Check sheet for the modelled part. Datum: model origin and axes. Units: mm. Coordinates: 2 decimals unless noted, no trailing zeros. Order: outer loops, then holes, each group sorted by start corner. A loop starts at its lowest first (then second) coordinate and runs counter-clockwise, first axis right, second up.
Autodesk Inventor part; units mm, degrees
ref_plane "YZ Plane" through (0, 0, 0) normal (1, 0, 0) x (0, 1, 0)
ref_plane "XZ Plane" through (0, 0, 0) normal (0, 1, 0) x (-1, 0, 0)
ref_plane "XY Plane" through (0, 0, 0) normal (0, 0, 1) x (1, 0, 0)
sketch "Sketch1" plane through (0, 0, 0) normal (1, 0, 0) x (0, 1, 0)
  line L0 (0, 80.1594) -> (0, -72.2406)
  circle A0 centre (101.6, 3.9594) radius 38.1
  line L1 (0, -72.2406) -> (114.2631, -31.9747)
  line L2 (0, 80.1594) -> (114.2631, 39.8934)
  point P0 (0, 0)
  dimension "d0" = 152.4
  dimension "d1" = 76.2
  dimension "d2" = 101.6
extrude "Extrusion1" add sketch "Sketch1" along normal blind 12.7
sketch "Sketch2" plane through (12.7, 0, 0) normal (1, 0, 0) x (0, 0, -1)
  arc A0 (31.9747, 114.2631) -> (-39.8934, 114.2631) centre (-3.9594, 101.6) ccw
  point P0 (0, 0)
hole "Hole1" at (12.7, 101.6, 3.9594) direction (-1, 0, 0) diameter 12.7 end through all
properties part number "Roller Frame"
(1) Cross-section at C-C (z = -11.5). Enter the section's corners in (x, y).
Filled in:
outline: (0, 0) - (12.7, 0) - (12.7, 136.42) - (0, 136.42) - close
(2) Go/stop test with flat-tipped pins: P1, Ø5, axis at x = 6, y = 31, coming from the +Z side; P2, Ø5, axis at x = 1.5, y = 19, coming from the +Z side; P3, Ø10, axis at y = 101.6, z = 3.96, coming from the +X side; P4, Ø1, axis at x = 3, y = 37, coming from the -Z side. Record where each tip stops, or that it passes through.
Filled in:
P1: stops at z = 70.12
P2: stops at z = 74.34
P3: passes through
P4: stops at z = -59.38
(3) Thickness scan on probe 1 along Z at (x, y) = (5.5, 101.6); probe 2 along Z at (x, y) = (2.25, 24); probe 3 along Y at (x, z) = (1, -5.5). Record the ranges inside material, lowest first.
Filled in:
probe 1: z = -36.44 to -2.39, 10.31 to 44.36
probe 2: z = -63.78 to 71.7
probe 3: y = 0 to 138.51
(4) Cross-section at B-B (x = 11). Enter the section's corners in (y, z), and give its area (3 significant figures).
Filled in:
outline: (0, -72.24) - (114.26, -31.97) arc R38.1 ccw to (114.26, 39.89) - (0, 80.16) - close; hole circle Ø12.7 at (101.6, 3.96)
area: 14,000 mm2
(5) Release check for a two-part mould opening along Z. For faces 1 (the cylindrical face through (6.261, 96.246, 0.546)), 2 (the flat face through (12.7, 53, 5)), 3 (the cylindrical face through (6.261, 139.694, 4.616)) record: +Z half, -Z half, draft (parallel to the pull), parting line (faces both ways), or undercut.
Filled in:
face 1: undercut
face 2: draft
face 3: parting line
(6) Cross-section at D-D (y = 84). Enter the section's corners in (x, z), and give its area (3 significant figures).
Filled in:
outline: (0, -42.64) - (12.7, -42.64) - (12.7, 50.56) - (0, 50.56) - close
area: 1,180 mm2
(7) Cross-section at A-A (y = 98.5). Enter the section's corners in (x, z), and give its area (3 significant figures).
Filled in:
outline: (0, -37.53) - (12.7, -37.53) - (12.7, -1.58) - (0, -1.58) - close; (0, 9.5) - (12.7, 9.5) - (12.7, 45.45) - (0, 45.45) - close
area: 913 mm2
